Input: part model. Units: mm. Frame: model coordinates. Face numbers are marked on the shaded views. A direction names the side the tool comes from. Round coordinates to 2 decimals unless told otherwise and drop trailing zeros. Order: outer loops, then holes, each group sorted by start corner. A loop starts at its lowest first (then second) coordinate and runs counter-clockwise, first axis right, second up. Notation, with made-up numbers: (24, 70.5) - (52, 70.5) arc R32 ccw to (52, 108.5) - close; hole circle Ø10 at (84, 58). An arc over 180 degrees is marked (long way). One line per item, written item: value. Start each with the question number.
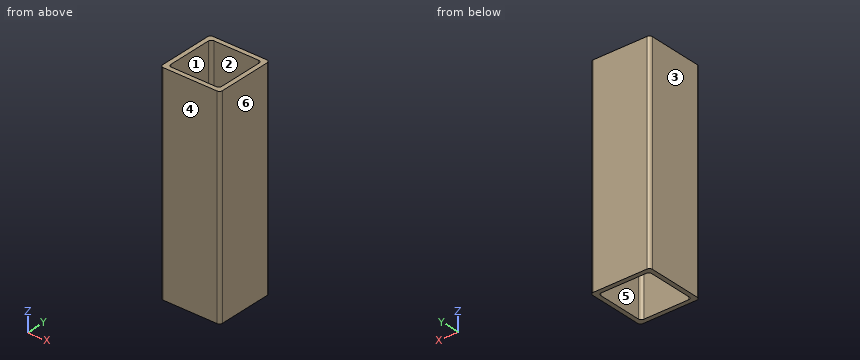
from build123d import *

# Parameters (mm, degrees)
SKETCH1_W           = 40
SKETCH1_H           = 40
BOSS_EXTRUDE1_DEPTH = 140
SKETCH2_W           = 34
SKETCH2_H           = 34
CUT_EXTRUDE1_DEPTH  = 143.828568571
FILLET1_R           = 2
FILLET2_R           = 2


with BuildPart() as part:
    # Sketch1 → Boss-Extrude1 (new body)
    with BuildSketch(Plane.XY):
        Rectangle(SKETCH1_W, SKETCH1_H)
    extrude(amount=BOSS_EXTRUDE1_DEPTH)

    # Sketch2 → Cut-Extrude1 (cut, through all)
    with BuildSketch(Plane.XY.offset(140)):
        Rectangle(SKETCH2_W, SKETCH2_H)
    extrude(amount=-CUT_EXTRUDE1_DEPTH, mode=Mode.SUBTRACT)

    # Fillet1
    fillet1_edges = [part.edges().sort_by_distance(p)[0] for p in [
        (20, -20, 70),
        (-20, -20, 70),
        (-20, 20, 70),
        (20, 20, 70),
    ]]
    fillet(fillet1_edges, radius=FILLET1_R)

    # Fillet2
    fillet2_edges = [part.edges().sort_by_distance(p)[0] for p in [
        (17, 17, 70),
        (17, -17, 70),
        (-17, -17, 70),
        (-17, 17, 70),
    ]]
    fillet(fillet2_edges, radius=FILLET2_R)


solid = part.part
1. Line query: line 1 (Y direction, x = 7.5, z = 33); line 2 (X direction, y = 15.5, z = 114.5). Output: solid intervals per line, ascending. Write a range as from..to.
2. Section C-C (z = 105). Return the cut outline in (x, y), then the cut area to 3 significant figures.
3. Pull-direction query (X, two-part tool) for the marked faces 1, 2, 3 and 4; classes: released by +X, released by -X, zero draft, split by the parting line, or undercut.
4. Set-up query: the marked faces 5 and 6. Return all of +Z, -Z, +X, -X, +Y, -Y with unobstructed straight access to the full face (end or side cutting, diameter ignored); none if empty.
5. Section A-A (y = 13.5). Return the cut outline in (x, z).
Solved:
1. line 1: y = -20..-17, 17..20
1. line 2: x = -20..-16.94, 16.94..20
2. outline: (-20, -18) arc R2 ccw to (-18, -20) - (18, -20) arc R2 ccw to (20, -18) - (20, 18) arc R2 ccw to (18, 20) - (-18, 20) arc R2 ccw to (-20, 18) - close; hole (-17, -15) arc R2 ccw to (-15, -17) - (15, -17) arc R2 ccw to (17, -15) - (17, 15) arc R2 ccw to (15, 17) - (-15, 17) arc R2 ccw to (-17, 15) - close
2. area: 444 mm²
3. face 1: undercut
3. face 2: undercut
3. face 3: released by -X
3. face 4: zero draft
4. face 5: +Z, -Z
4. face 6: +Z, -Z, +X, +Y, -Y
5. outline: (-20, 0) - (-17, 0) - (-17, 140) - (-20, 140) - close; (17, 0) - (20, 0) - (20, 140) - (17, 140) - close
